from build123d import *

# Parameters (mm, degrees)
ESQUISSE1_W      = 71
ESQUISSE1_H      = 37.6
EXTRUSION1_DEPTH = 18.8
CONG_1_R         = 4
CONG_2_R         = 4
CONG_3_R         = 4


with BuildPart() as part:
    # Esquisse1 → Extrusion1 (new body)
    with BuildSketch(Plane.XY):
        with Locations((-7.553014699, -1.477523911)):
            Rectangle(ESQUISSE1_W, ESQUISSE1_H)
    extrude(amount=EXTRUSION1_DEPTH)

    # Congé1
    cong_1_edges = [part.edges().sort_by_distance(p)[0] for p in [
        (-7.553014699, 17.322476089, 18.8),
    ]]
    fillet(cong_1_edges, radius=CONG_1_R)

    # Congé2
    cong_2_edges = [part.edges().sort_by_distance(p)[0] for p in [
        (-7.553014699, -20.277523911, 18.8),
        (-7.553014699, 17.322476089, 0),
    ]]
    fillet(cong_2_edges, radius=CONG_2_R)

    # Congé3
    cong_3_edges = [part.edges().sort_by_distance(p)[0] for p in [
        (-7.553014699, -20.277523911, 0),
    ]]
    fillet(cong_3_edges, radius=CONG_3_R)


solid = part.part
Check sheet for the modelled part. Datum: model origin and axes. Units: mm. Coordinates: 2 decimals unless noted, no trailing zeros. Loops run counter-clockwise (first coordinate to the right, second up) from the corner with the lowest first, then second, coordinate; pieces in that order, holes last. Notation, with made-up numbers: (33.5, -7.75) -> (80.5, -7.75) arc R20 ccw to (80.5, 17.25) -> close; hole circle Ø5 at (23, -34.75). An arc over 180 degrees is marked (long way). Write item = value, one per line. Start each with the question number.
1. Section check A-A on x = -18.5. Record the cut outline in (y, z).
2. Section check B-B on y = 14.5. Record the cut outline in (x, z), then the cut area to 3 significant figures.
3. Depth check by flat-ended pin: P1, Ø5, axis at x = -10.5, z = 16, coming from the -Y side. Enter the tip coordinate at first touch or a pass-through.
4. Material ranges on line 1 (Z direction, x = -10, y = 15.5); line 2 (Z direction, x = -20, y = 14); line 3 (Y direction, x = -1.5, z = 16), recorded low to high.
Responses:
q1.outline = (-20.28, 4) arc R4 ccw to (-16.28, 0) -> (13.32, 0) arc R4 ccw to (17.32, 4) -> (17.32, 14.8) arc R4 ccw to (13.32, 18.8) -> (-16.28, 18.8) arc R4 ccw to (-20.28, 14.8) -> close
q2.outline = (-43.05, 0.18) -> (27.95, 0.18) -> (27.95, 18.62) -> (-43.05, 18.62) -> close
q2.area = 1,310 mm2
q3.P1 = -20.28
q4.line_1 = 0.64 to 18.16
q4.line_2 = 0.06 to 18.74
q4.line_3 = -20.09 to 17.14
